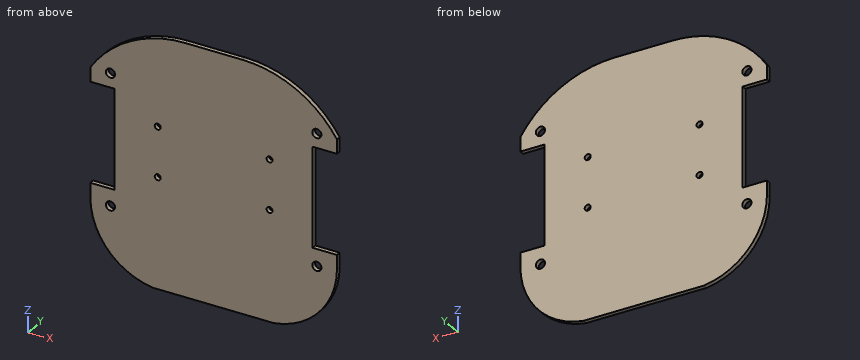
Autodesk Inventor part; units mm, degrees
ref_plane "YZ Plane" through (0, 0, 0) normal (1, 0, 0) x (0, 1, 0)
ref_plane "XZ Plane" through (0, 0, 0) normal (0, 1, 0) x (-1, 0, 0)
ref_plane "XY Plane" through (0, 0, 0) normal (0, 0, 1) x (1, 0, 0)
sketch "Esquisse1" plane through (0, 0, 0) normal (0, 1, 0) x (-1, 0, 0)
  line L0 (-43, -44) -> (43, -44)
  line L1 (43, -44) -> (43, 44)
  line L2 (43, 44) -> (-43, 44)
  line L3 (-43, 44) -> (-43, -44)
  point P0 (0, 0)
  dimension "d0" = 86
  dimension "d1" = 88
  dimension "d2" = 43
  dimension "d3" = 44
extrude "Carre de base" add sketch "Esquisse1" along normal blind 1.6
sketch "Esquisse2" plane through (0, 1.6, 0) normal (0, 1, 0) x (1, 0, 0)
  line L0 (43, 44) -> (-43, 44)
  line L1 (-43, 44) -> (-43, -44)
  line L2 (-43, -44) -> (43, -44)
  line L3 (43, -44) -> (43, 44)
  line L4 (-43, 14) -> (-34.5, 14)
  line L5 (-34.5, 14) -> (-34.5, -21)
  line L6 (-34.5, -21) -> (-43, -21)
  line L7 (43, 14) -> (34.5, 14)
  line L8 (34.5, 14) -> (34.5, -21)
  line L9 (34.5, -21) -> (43, -21)
  line L10 (-43, -21) -> (-43, -26)
  line L11 (43, -21) -> (43, -26)
  line L12 (-43, 14) -> (-43, 19)
  line L13 (43, 14) -> (43, 19)
  line L14 (10, -44) -> (-10, -44)
  line L15 (21, 44) -> (-21, 44)
  arc A0 (10, -44) -> (43, -26) centre (10, -4.75) ccw
  arc A1 (-43, -26) -> (-10, -44) centre (-10, -4.75) ccw
  arc A2 (43, 19) -> (21, 44) centre (17.7955, 19) ccw
  arc A3 (-21, 44) -> (-43, 19) centre (-17.7955, 19) ccw
  point P0 (0, 0)
  dimension "d6" = 35
  dimension "d7" = 30
  dimension "d8" = 30
  dimension "d9" = 8.5
  dimension "d10" = 8.5
  dimension "d11" = 35
  dimension "d13" = 5
  dimension "d14" = 5
  dimension "d15" = 5
  dimension "d16" = 5
  dimension "d21" = 20
  dimension "d22" = 10
  dimension "d23" = 42
  dimension "d24" = 21
  dimension "d25" = 39.25
  dimension "d26" = 39.25
  dimension "d27" = 25.2046
  dimension "d28" = 25.2046
extrude "Evidement" cut sketch "Esquisse2" against normal through all contours L3 A2 L0 | A3 L1 L0 | L3 L9 L8 L7 | L4 L5 L6 L1 | L3 L2 A0 | A1 L2 L1
sketch "Esquisse3" plane through (0, 1.6, 0) normal (0, 1, 0) x (1, 0, 0)
  line L0 (34.5, -21) -> (34.5, 14)
  line L1 (-34.5, 14) -> (-34.5, -21)
  circle A0 centre (-19.5, 5.25) radius 1.05
  circle A1 centre (-19.5, -12.25) radius 1.05
  circle A2 centre (19.5, 5.25) radius 1.05
  circle A3 centre (19.5, -12.25) radius 1.05
  point P0 (0, 0)
  dimension "d31" = 2.1
  dimension "d32" = 17.5
  dimension "d33" = 2.1
  dimension "d34" = 2.1
  dimension "d35" = 2.1
  dimension "d36" = 17.5
  dimension "d37" = 15
  dimension "d38" = 15
  dimension "d39" = 15
  dimension "d40" = 15
  dimension "d41" = 35
  dimension "d42" = 8.75
  dimension "d43" = 8.75
extrude "Extrusion4" cut sketch "Esquisse3" against normal through all
sketch "Esquisse6" plane through (0, 0, 0) normal (0, -1, 0) x (1, 0, 0)
  circle A0 centre (-36, 26) radius 1.6
  circle A1 centre (36, 26) radius 1.6
  circle A2 centre (36, -20) radius 1.6
  circle A3 centre (-36, -20) radius 1.6
  point P0 (0, 0)
  dimension "d59" = 36
  dimension "d60" = 36
  dimension "d61" = 36
  dimension "d62" = 36
  dimension "d63" = 26
  dimension "d64" = 26
  dimension "d65" = 20
  dimension "d66" = 20
  dimension "d67" = 3.2
  dimension "d68" = 3.2
  dimension "d69" = 3.2
  dimension "d70" = 3.2
extrude "Extrusion7" cut sketch "Esquisse6" against normal through all
equation "\"d8\" = d7"
equation "\"d9\" = d10"
equation "\"d11\" = d6"
equation "\"d13\" = d14"
equation "\"d15\" = d16"
equation "\"d26\" = d25"
equation "\"d28\" = d27"
equation "\"d33\" = d31"
equation "\"d34\" = d31"
equation "\"d35\" = d31"
equation "\"d36\" = d32"
equation "\"d38\" = d37"
equation "\"d39\" = d37"
equation "\"d40\" = d37"
equation "\"d42\" = -0.5 * d36 + 0.5 * d41"
equation "\"d43\" = d42"
equation "\"d68\" = d67"
equation "\"d69\" = d67"
equation "\"d70\" = d67"
properties part number "pcb"
The listing builds one solid part. Answer for the finished solid, in the listing's coordinates (mm). Round coordinates to 2 decimals unless told otherwise and drop trailing zeros. Loops run counter-clockwise (first coordinate to the right, second up) from the corner with the lowest first, then second, coordinate; pieces in that order, holes last. Notation, with made-up numbers: M -17,40.25 L 33,40.25 A18 cw 33,57.25 Z; hole C 58.5,-0.5 d9. An arc over 180 degrees is marked long. Return JSON: item names as keys, results as strings.
Q1. Find section C-C, the plane x = -19.5. Determine the outline of the cut face in (y, z).
Results list:
{"outline": "M 0,-44 L 1.6,-44 L 1.6,-6.3 L 0,-6.3 Z; M 0,-4.2 L 1.6,-4.2 L 1.6,11.2 L 0,11.2 Z; M 0,13.3 L 1.6,13.3 L 1.6,42.83 L 0,42.83 Z"}
Q2. Find the intervals of material crossed by line 1 along X through (y, z) = (0.9, 12.25); line 2 along Z through (x, y) = (19.5, 0.6); line 3 along Z through (x, y) = (36, 0.65), in increasing order. Write a range as from..to.
Results list:
{"line 1": "x = -34.5..-20.55, -18.45..18.45, 20.55..34.5", "line 2": "z = -44..-6.3, -4.2..11.2, 13.3..42.83", "line 3": "z = -36.43..-21.6, -18.4..-14, 21..24.4, 27.6..34.15"}
Q3. Find section B-B, the plane z = -5.25. Determine the outline of the cut face in (x, y), plus the area to 3 significant figures.
Results list:
{"outline": "M -34.5,0 L -20.55,0 L -20.55,1.6 L -34.5,1.6 Z; M -18.45,0 L 18.45,0 L 18.45,1.6 L -18.45,1.6 Z; M 20.55,0 L 34.5,0 L 34.5,1.6 L 20.55,1.6 Z", "area": "104 mm2"}
Q4. Each of these flat-tipped pins is pushed along its axis until it touches: pin 1 Ø0.5 at (y, z) = (1, 3) entering from +X; pin 2 Ø1.9 at (x, z) = (-36, 26) entering from +Y; pin 3 Ø2.5 at (x, z) = (19.5, 12.25) entering from -Y; pin 4 Ø0.5 at (x, y) = (-38, 0.5) entering from -Z. Where does it stop, or does it pass through?
Results list:
{"pin 1": "stops at x = 34.5", "pin 2": "passes through", "pin 3": "stops at y = 0", "pin 4": "stops at z = -34.4"}
Q5. Find section A-A, the plane y = 0.5. State how many separate pieces and enclosed holes the cut face has, plus the area to 3 significant figures.
Results list:
{"separate pieces": "1", "enclosed holes": "8", "area": "6,310 mm2"}
Q6. Find section D-D, the plane x = -36. Determine the outline of the cut face in (y, z), plus the area to 3 significant figures.
Results list:
{"outline": "M 0,-36.43 L 1.6,-36.43 L 1.6,-21.6 L 0,-21.6 Z; M 0,-18.4 L 1.6,-18.4 L 1.6,-14 L 0,-14 Z; M 0,21 L 1.6,21 L 1.6,24.4 L 0,24.4 Z; M 0,27.6 L 1.6,27.6 L 1.6,34.15 L 0,34.15 Z", "area": "46.7 mm2"}
